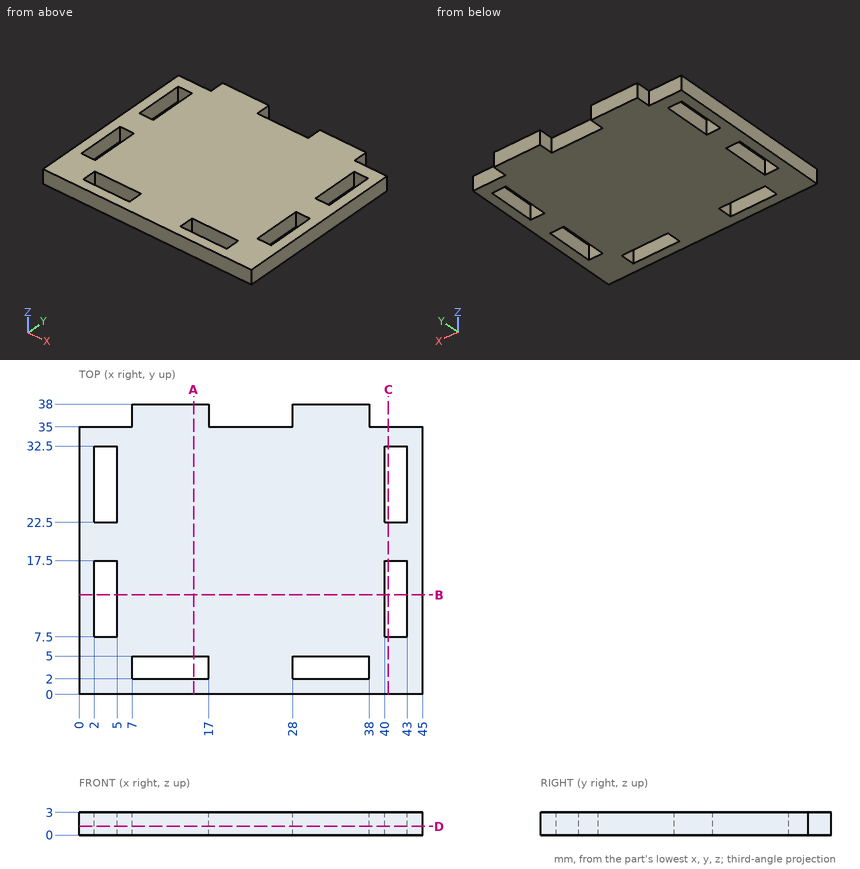
Job drawing, mm, ordinate dimensions from the low corner. One solid piece. Round coordinates to 2 decimals unless told otherwise and drop trailing zeros. Loops run counter-clockwise (first coordinate to the right, second up) from the corner with the lowest first, then second, coordinate; pieces in that order, holes last. Notation, with made-up numbers: (81.5, -2.75) -> (88.5, -2.75) arc R6 ccw to (88.5, 6.25) -> close; hole circle Ø1 at (39, 83). An arc over 180 degrees is marked (long way). Use a Markdown table: item, result.
1) Cut at B-B, the plane y = 13. List the corners of the cut face in (x, z).
The answers:
| item | result |
|---|---|
| outline | (0, 0) -> (2, 0) -> (2, 3) -> (0, 3) -> close; (5, 0) -> (40, 0) -> (40, 3) -> (5, 3) -> close; (43, 0) -> (45, 0) -> (45, 3) -> (43, 3) -> close |
2) Drop flat-ended pins along their axis: pin 1 Ø0.9 at (y, z) = (26.5, 1.5) entering from -X; pin 2 Ø1.5 at (x, z) = (40, 2) entering from +Y. Give the stop position or say it passes through.
The answers:
| item | result |
|---|---|
| pin 1 | stops at x = 0 |
| pin 2 | stops at y = 35 |
3) Probe line 1 (X direction, y = 27, z = 1); line 2 (Y direction, x = 2.5, z = 2.95); line 3 (Y direction, x = 28.5, z = 0.3). List the from-to ranges inside material, lowest first. Write a range as [from, to].
The answers:
| item | result |
|---|---|
| line 1 | x = [0, 2], [5, 40], [43, 45] |
| line 2 | y = [0, 7.5], [17.5, 22.5], [32.5, 35] |
| line 3 | y = [0, 2], [5, 38] |
4) Cut at D-D, the plane z = 1.15. State how many separate pieces and enclosed holes the cut face has, and give its area (4 significant figures).
The answers:
| item | result |
|---|---|
| separate pieces | 1 |
| enclosed holes | 6 |
| area | 1,455 mm2 |
5) Cut at A-A, the plane x = 15. List the corners of the cut face in (y, z).
The answers:
| item | result |
|---|---|
| outline | (0, 0) -> (2, 0) -> (2, 3) -> (0, 3) -> close; (5, 0) -> (38, 0) -> (38, 3) -> (5, 3) -> close |
6) Cut at C-C, the plane x = 40.5. List the corners of the cut face in (y, z).
The answers:
| item | result |
|---|---|
| outline | (0, 0) -> (7.5, 0) -> (7.5, 3) -> (0, 3) -> close; (17.5, 0) -> (22.5, 0) -> (22.5, 3) -> (17.5, 3) -> close; (32.5, 0) -> (35, 0) -> (35, 3) -> (32.5, 3) -> close |
